Geometry check sheet. Reference: the model listing, model coordinates, mm. Give positions to 0.01 mm unless a question says otherwise; leave off trailing zeros. Write each loop counter-clockwise with the first axis right and the second up, starting at its lowest first coordinate (ties: lowest second). Pieces come first, ordered by that corner, then holes. Notation, with made-up numbers: (78.25, 71.25) -> (98.25, 71.25) arc R12 cw to (98.25, 91.25) -> close; hole circle Ø4 at (32.5, 25.5). An arc over 180 degrees is marked (long way). One line per item, written item: value.
Autodesk Inventor part; units mm, degrees
ref_plane "YZ Plane" through (0, 0, 0) normal (1, 0, 0) x (0, 1, 0)
ref_plane "XZ Plane" through (0, 0, 0) normal (0, 1, 0) x (-1, 0, 0)
ref_plane "XY Plane" through (0, 0, 0) normal (0, 0, 1) x (1, 0, 0)
sketch "Sketch1" plane through (0, 0, 0) normal (0, 1, 0) x (-1, 0, 0)
  circle A0 centre (0, 0) radius 35
  circle A1 centre (0, 0) radius 25
  dimension "d1" = 70
  dimension "d2" = 50
sketch "Sketch2" plane through (0, 0, 0) normal (0, 1, 0) x (-1, 0, 0)
  circle A0 centre (0, 0) radius 25
  circle A1 centre (0, 0) radius 35
  dimension "d3" = 50
  dimension "d4" = 70
extrude "Extrusion1" add sketch "Sketch1" along normal blind 7
extrude "Extrusion2" add sketch "Sketch2" along normal blind 13 contours A0
sketch "Sketch3" plane through (0, 0, 0) normal (0, -1, 0) x (1, 0, 0)
  line L0 (0, 0) -> (0, -35)
  circle A0 centre (0, 0) radius 35
  line L1 (0, 35) -> (0, 0)
  line L2 (30.3109, -17.5) -> (0, -35)
  line L3 (0, -35) -> (-30.3109, -17.5)
  line L4 (-30.3109, -17.5) -> (-30.3109, 17.5)
  line L5 (-30.3109, 17.5) -> (0, 35)
  line L6 (0, 35) -> (30.3109, 17.5)
  line L7 (30.3109, 17.5) -> (30.3109, -17.5)
  line L8 (0, 0) -> (30.3109, 17.5)
  line L9 (0, 0) -> (0, 35)
  line L10 (0, 0) -> (-30.3109, 17.5)
  line L11 (0, 0) -> (-30.3109, -17.5)
  line L12 (0, 0) -> (0, -35)
  line L13 (0, 0) -> (30.3109, -17.5)
  line L14 (30.3109, 17.5) -> (26.8468, 15.5)
  line L15 (26.8468, 15.5) -> (26.8468, -15.5)
  line L16 (0, -35) -> (0, -31)
  line L17 (-30.3109, -17.5) -> (-26.8468, -15.5)
  line L18 (0, 35) -> (0, 31)
  line L19 (-30.3109, 17.5) -> (-26.8468, 15.5)
  dimension "d9" = 4
  dimension "d10" = 4
  dimension "d11" = 4
  dimension "d12" = 4
  dimension "d13" = 4
hole "Hole1" at (26.8468, 0, 15.5) at (26.8468, 0, -15.5) at (0, 0, -31) at (-26.8468, 0, -15.5) at (-26.8468, 0, 15.5) at (0, 0, 31) direction (0, 1, 0) diameter 3 end through all
properties part number "bat_endcap"
1) Mould release check, pull along X, two halves, no side actions. Record for faces 1 (the cylindrical face through (-23.846, 9.958, -7.509)), 2 (the flat face through (-10.2, 7, -23.2)), 3 (the cylindrical face through (25.833, 3.549, 16.606)): released by +X, released by -X, zero draft, split by the parting line, or undercut.
Verdict:
face 1: split by the parting line
face 2: zero draft
face 3: undercut
2) Scan lines: probe 1 along X at (y, z) = (3, 15.5); probe 2 along Z at (x, y) = (-25.5, 2.5); probe 3 along Z at (x, y) = (-26, 4). Record each from-to range of solid material in increasing order.
Verdict:
probe 1: -31.38 to -28.35, -25.35 to 25.35, 28.35 to 31.38
probe 2: -23.97 to -16.16, -14.84 to 14.84, 16.16 to 23.97
probe 3: -23.43 to -16.74, -14.26 to 14.26, 16.74 to 23.43
3) Sectioned sample at B-B on z = -15.5. Record the cut outline in (x, y), plus the area to 3 significant figures.
Verdict:
outline: (-31.38, 0) -> (-28.35, 0) -> (-28.35, 7) -> (-31.38, 7) -> close; (-25.35, 0) -> (25.35, 0) -> (25.35, 7) -> (19.62, 7) -> (19.62, 13) -> (-19.62, 13) -> (-19.62, 7) -> (-25.35, 7) -> close; (28.35, 0) -> (31.38, 0) -> (31.38, 7) -> (28.35, 7) -> close
area: 633 mm^2
4) Depth check by flat-ended pin: pin 1 Ø1.5 at (y, z) = (3.5, 10) entering from +X; pin 2 Ø2.5 at (x, z) = (0, 31) entering from -Y; pin 3 Ø1 at (y, z) = (1.5, 25) entering from -X (3 decimals); pin 4 Ø1.5 at (x, y) = (-17, 7.5) entering from -Z. Enter the tip coordinate at first touch or a pass-through.
Verdict:
pin 1: x = 33.76
pin 2: through
pin 3: x = -24.995
pin 4: z = -30.9
5) Sectioned sample at C-C on z = -31. Record the cut outline in (x, y).
Verdict:
outline: (-16.25, 0) -> (-1.5, 0) -> (-1.5, 7) -> (-16.25, 7) -> close; (1.5, 0) -> (16.25, 0) -> (16.25, 7) -> (1.5, 7) -> close
6) Sectioned sample at D-D on y = 5.5. Record the cut outline in (x, z), plus the area to 3 significant figures.
Verdict:
outline: circle Ø70 at (0, 0); hole circle Ø3 at (-26.85, -15.5); hole circle Ø3 at (-26.85, 15.5); hole circle Ø3 at (0, -31); hole circle Ø3 at (0, 31); hole circle Ø3 at (26.85, -15.5); hole circle Ø3 at (26.85, 15.5)
area: 3,810 mm^2
7) Sectioned sample at A-A on x = 0. Record the cut outline in (y, z), plus the area to 3 significant figures.
Verdict:
outline: (0, -35) -> (7, -35) -> (7, -32.5) -> (0, -32.5) -> close; (0, -29.5) -> (7, -29.5) -> (7, -25) -> (13, -25) -> (13, 25) -> (7, 25) -> (7, 29.5) -> (0, 29.5) -> close; (0, 32.5) -> (7, 32.5) -> (7, 35) -> (0, 35) -> close
area: 748 mm^2
